from build123d import *

# Parameters (mm, degrees)
SKETCH1_R           = 5.5
BOSS_EXTRUDE1_DEPTH = 0.6
SKETCH2_R           = 5
BOSS_EXTRUDE2_DEPTH = 3
SKETCH3_R           = 3
CUT_EXTRUDE1_DEPTH  = 9.570880935
SKETCH4_R           = 4.75
SKETCH4_R_2         = 4.375
CUT_EXTRUDE2_DEPTH  = 0.25
FILLET1_R           = 0.25
FILLET2_R           = 0.25


with BuildPart() as part:
    # Sketch1 → Boss-Extrude1 (new body)
    with BuildSketch(Plane(origin=(0, 0, 0), x_dir=(0, 0, -1), z_dir=(1, 0, 0))):
        Circle(SKETCH1_R)
    extrude(amount=BOSS_EXTRUDE1_DEPTH)

    # Sketch2 → Boss-Extrude2 (add)
    with BuildSketch(Plane(origin=(0.6, 0, 0), x_dir=(0, 0, -1), z_dir=(1, 0, 0))):
        Circle(SKETCH2_R)
    extrude(amount=BOSS_EXTRUDE2_DEPTH)

    # Sketch3 → Cut-Extrude1 (cut, through all)
    with BuildSketch(Plane(origin=(3.6, 0, 0), x_dir=(0, 0, -1), z_dir=(1, 0, 0))):
        Circle(SKETCH3_R)
    extrude(amount=-CUT_EXTRUDE1_DEPTH, mode=Mode.SUBTRACT)

    # Sketch4 → Cut-Extrude2 (cut)
    with BuildSketch(Plane.ZY):
        Circle(SKETCH4_R)
        Circle(SKETCH4_R_2, mode=Mode.SUBTRACT)
    extrude(amount=-CUT_EXTRUDE2_DEPTH, mode=Mode.SUBTRACT)

    # Fillet1
    fillet1_edges = [part.edges().sort_by_distance(p)[0] for p in [
        (0, 0, 5.5),
    ]]
    fillet(fillet1_edges, radius=FILLET1_R)

    # Fillet2
    fillet2_edges = [part.edges().sort_by_distance(p)[0] for p in [
        (3.6, 0, 5),
    ]]
    fillet(fillet2_edges, radius=FILLET2_R)


solid = part.part
The model under review builds one solid part; all positions refer to its coordinate system, in mm. A direction names the side the tool comes from. Coordinates: 2 decimals unless noted, no trailing zeros. Loops run counter-clockwise (first coordinate to the right, second up) from the corner with the lowest first, then second, coordinate; pieces in that order, holes last.
(1) Consider section A-A, the plane y = 0. Give the boundary of the cut face in (x, z) (3 decimals).
Determined:
outline: (0, -5.25) arc R0.25 ccw to (0.25, -5.5) - (0.6, -5.5) - (0.6, -5) - (3.35, -5) arc R0.25 ccw to (3.6, -4.75) - (3.6, -3) - (0, -3) - (0, -4.375) - (0.25, -4.375) - (0.25, -4.75) - (0, -4.75) - close; (0, 3) - (3.6, 3) - (3.6, 4.75) arc R0.25 ccw to (3.35, 5) - (0.6, 5) - (0.6, 5.5) - (0.25, 5.5) arc R0.25 ccw to (0, 5.25) - (0, 4.75) - (0.25, 4.75) - (0.25, 4.375) - (0, 4.375) - close
(2) Consider section C-C, the plane x = 1.9. Give the boundary of the cut face in (y, z).
Determined:
outline: circle Ø10 at (0, 0); hole circle Ø6 at (0, 0)
(3) Draft analysis for pull direction Z (two halves, no side actions). For faces 1 (the flat face through (0.6, -4.9, -1.6)), 2 (the cylindrical face through (0.42, -5.37, 1.19)), 3 (the cylindrical face through (2, 0, 3)), state which applies: +Z half, -Z half, draft (parallel to the pull), parting line (faces both ways), or undercut.
Determined:
face 1: draft
face 2: parting line
face 3: undercut
(4) Tool access review of faces 4 (the cylindrical face through (1.96, -4.88, 1.08)), 5 (the flat face through (0, -3, 4)): name each direction out of +Z, -Z, +X, -X, +Y, -Y from which nothing blocks a thin tool from reaching the whole face with its end or side.
Determined:
face 4: +X
face 5: +Z, -Z, -X, +Y, -Y
(5) Wall thickness on L1, parallel to Y at x = 2.55, z = 0; L2, parallel to Z at x = 2.45, y = 2.5; L3, parallel to Z at x = 0.5, y = -2.5: over which ranges is each line inside the solid? List them lowest first.
Determined:
L1: y = -5 to -3, 3 to 5
L2: z = -4.33 to -1.66, 1.66 to 4.33
L3: z = -4.9 to -1.66, 1.66 to 4.9
(6) Insertion check: P1, Ø2, axis at x = 2, y = -3, coming from the +Z side; P2, Ø1.5, axis at x = 2, y = -3, coming from the -Z side; P3, Ø3.5, axis at y = 2, z = -0.5, coming from the +X side; P4, Ø1, axis at x = 1.5, y = -2.5, coming from the -Z side. Each pin has a flat end and moves straight along its axis. Give the tip position at first contact, or say it passes through.
Determined:
P1: stops at z = 4.58
P2: stops at z = -4.47
P3: stops at x = 3.6
P4: stops at z = -4.58
